```python
from build123d import *

# Parameters (mm, degrees)
SKETCH1_R               = 8
SKETCH1_R_2             = 10
SKETCH1_R_3             = 1.25
SKETCH1_R_4             = 1.5
SKETCH1_R_5             = 1.8
BOSS_EXTRUDE1_DEPTH     = 6
FILLET1_R               = 10
SKETCH2_W               = 15
SKETCH2_H               = 22
BOSS_EXTRUDE2_DEPTH     = 6
SKETCH3_R               = 1
CUT_EXTRUDE1_DEPTH      = 159.031622895
CHAMFER1_SIZE           = 1
MOVE_FACE1_OUTLINE_R    = 8
MOVE_FACE1_OUTLINE_R_2  = 7.92
MOVE_FACE1_OUTLINE_R_3  = 10
MOVE_FACE1_OUTLINE_R_4  = 9.92
MOVE_FACE1_OUTLINE_R_5  = 1.25
MOVE_FACE1_OUTLINE_R_6  = 1.17
MOVE_FACE1_OUTLINE_R_7  = 1.5
MOVE_FACE1_OUTLINE_R_8  = 1.42
MOVE_FACE1_OUTLINE_R_9  = 1.8
MOVE_FACE1_OUTLINE_R_10 = 1.72
MOVE_FACE1_DEPTH        = 6


# Read off the part's stored shape, not the designer's step: Move Face1
with BuildPart() as part:
    # Sketch1 → Boss-Extrude1 (new body)
    with BuildSketch(Plane.XY):
        with BuildLine():
            Line((-40.498784978, 0), (0, 0))
            Line((0, 0), (0, 75))
            ThreePointArc((0, 75), (-37.5, 112.5), (-75, 75))
            Line((-75, 75), (-75, 55))
            Line((-75, 55), (-83.323029145, 55))
            ThreePointArc((-83.323029145, 55), (-110.823029145, 27.5), (-83.323029145, 0))
            Line((-83.323029145, 0), (-40.498784978, 0))
        make_face()
        with Locations((-83.323029145, 27.5)):
            Circle(SKETCH1_R, mode=Mode.SUBTRACT)
        with Locations((-37.5, 75)):
            Circle(SKETCH1_R_2, mode=Mode.SUBTRACT)
        with Locations((-83.323029145, 50.5)):
            Circle(SKETCH1_R_3, mode=Mode.SUBTRACT)
        with Locations((-67.059573177, 43.763455967)):
            Circle(SKETCH1_R_4, mode=Mode.SUBTRACT)
        with Locations((-60.323029145, 27.5)):
            Circle(SKETCH1_R_3, mode=Mode.SUBTRACT)
        with Locations((-67.059573177, 11.236544033)):
            Circle(SKETCH1_R_4, mode=Mode.SUBTRACT)
        with Locations((-83.323029145, 4.5)):
            Circle(SKETCH1_R_3, mode=Mode.SUBTRACT)
        with Locations((-37.5, 102.5)):
            Circle(SKETCH1_R_5, mode=Mode.SUBTRACT)
        with Locations((-65, 75)):
            Circle(SKETCH1_R_5, mode=Mode.SUBTRACT)
        with Locations((-10, 75)):
            Circle(SKETCH1_R_5, mode=Mode.SUBTRACT)
        with Locations((-37.5, 47.5)):
            Circle(SKETCH1_R_5, mode=Mode.SUBTRACT)
        with Locations((-56.945436483, 94.445436483)):
            Circle(SKETCH1_R_4, mode=Mode.SUBTRACT)
        with Locations((-18.054563517, 94.445436483)):
            Circle(SKETCH1_R_4, mode=Mode.SUBTRACT)
        with Locations((-18.054563517, 55.554563517)):
            Circle(SKETCH1_R_4, mode=Mode.SUBTRACT)
        with Locations((-56.945436483, 55.554563517)):
            Circle(SKETCH1_R_4, mode=Mode.SUBTRACT)
        with Locations((-37.5, 88)):
            Circle(SKETCH1_R_5, mode=Mode.SUBTRACT)
        with Locations((-24.5, 75)):
            Circle(SKETCH1_R_5, mode=Mode.SUBTRACT)
        with Locations((-37.5, 62)):
            Circle(SKETCH1_R_5, mode=Mode.SUBTRACT)
        with Locations((-50.5, 75)):
            Circle(SKETCH1_R_5, mode=Mode.SUBTRACT)
    extrude(amount=BOSS_EXTRUDE1_DEPTH)

    # Fillet1
    fillet1_edges = [part.edges().sort_by_distance(p)[0] for p in [
        (-75, 55, 3),
    ]]
    fillet(fillet1_edges, radius=FILLET1_R)

    # Sketch2 → Boss-Extrude2 (add)
    with BuildSketch(Plane(origin=(0, 0, 0), x_dir=(-1, 0, 0), z_dir=(0, 0, -1))):
        with Locations((7.5, -11)):
            Rectangle(SKETCH2_W, SKETCH2_H)
        with Locations((37.5, -11)):
            Rectangle(SKETCH2_W, SKETCH2_H)
        with Locations((67.5, -11)):
            Rectangle(SKETCH2_W, SKETCH2_H)
    extrude(amount=-BOSS_EXTRUDE2_DEPTH)

    # Sketch3 → Cut-Extrude1 (cut, through all)
    with BuildSketch(Plane.XY.offset(6)):
        with Locations((-75, 0)):
            Circle(SKETCH3_R)
        with Locations((-60, 0)):
            Circle(SKETCH3_R)
        with Locations((-45, 0)):
            Circle(SKETCH3_R)
        with Locations((-30, 0)):
            Circle(SKETCH3_R)
        with Locations((-15, 0)):
            Circle(SKETCH3_R)
    extrude(amount=-CUT_EXTRUDE1_DEPTH, mode=Mode.SUBTRACT)

    # Chamfer1
    chamfer1_edges = [part.edges().sort_by_distance(p)[0] for p in [
        (0, -22, 3),
        (-15, -22, 3),
        (-30, -22, 3),
        (-45, -22, 3),
        (-60, -22, 3),
        (-75, -22, 3),
    ]]
    chamfer(chamfer1_edges, length=CHAMFER1_SIZE)

    # Move Face1 outline → Move Face1 (add)
    # profile 1 of 24: a face of its own
    with BuildSketch(Plane.XY):
        with BuildLine():
            Line((-59.003205136, -0.08), (-45.996794864, -0.08))
            ThreePointArc((-45.996794864, -0.08), (-45.999198395, -0.04003209), (-46, 0))
            Line((-46, 0), (-59, 0))
            ThreePointArc((-59, 0), (-59.000801605, -0.04003209), (-59.003205136, -0.08))
        make_face()
    # profile 2 of 24: a face of its own
    with BuildSketch(Plane.XY):
        with BuildLine():
            Line((-45, -21), (-45, -1))
            ThreePointArc((-45, -1), (-45.04003209, -0.999198395), (-45.08, -0.996794864))
            Line((-45.08, -0.996794864), (-45.08, -21.033137085))
            Line((-45.08, -21.033137085), (-44.033137085, -22.08))
            Line((-44.033137085, -22.08), (-30.966862915, -22.08))
            Line((-30.966862915, -22.08), (-29.92, -21.033137085))
            Line((-29.92, -21.033137085), (-29.92, -0.996794864))
            ThreePointArc((-29.92, -0.996794864), (-29.95996791, -0.999198395), (-30, -1))
            Line((-30, -1), (-30, -21))
            Line((-30, -21), (-31, -22))
            Line((-31, -22), (-44, -22))
            Line((-44, -22), (-45, -21))
        make_face()
    # profile 3 of 24: a face of its own
    with BuildSketch(Plane.XY):
        with BuildLine():
            ThreePointArc((-59.92, -0.996794864), (-59.95996791, -0.999198395), (-60, -1))
            Line((-60, -1), (-60, -21))
            Line((-60, -21), (-61, -22))
            Line((-61, -22), (-74, -22))
            Line((-74, -22), (-75, -21))
            Line((-75, -21), (-75, -1))
            ThreePointArc((-75, -1), (-75.04003209, -0.999198395), (-75.08, -0.996794864))
            Line((-75.08, -0.996794864), (-75.08, -21.033137085))
            Line((-75.08, -21.033137085), (-74.033137085, -22.08))
            Line((-74.033137085, -22.08), (-60.966862915, -22.08))
            Line((-60.966862915, -22.08), (-59.92, -21.033137085))
            Line((-59.92, -21.033137085), (-59.92, -0.996794864))
        make_face()
    # profile 4 of 24: a face of its own
    with BuildSketch(Plane.XY):
        with BuildLine():
            Line((-16, 0), (-29, 0))
            ThreePointArc((-29, 0), (-29.000801605, -0.04003209), (-29.003205136, -0.08))
            Line((-29.003205136, -0.08), (-15.996794864, -0.08))
            ThreePointArc((-15.996794864, -0.08), (-15.999198395, -0.04003209), (-16, 0))
        make_face()
    # profile 5 of 24: a face of its own
    with BuildSketch(Plane.XY):
        with BuildLine():
            ThreePointArc((-75.996794864, -0.08), (-75.999198395, -0.04003209), (-76, 0))
            Line((-76, 0), (-83.323029145, 0))
            ThreePointArc((-83.323029145, 0), (-110.816150501, 26.884956844), (-84.552807772, 54.972488867))
            ThreePointArc((-84.552807772, 54.972488867), (-77.772555006, 58.051331596), (-75, 64.962484818))
            Line((-75, 64.962484818), (-75, 75))
            ThreePointArc((-75, 75), (-37.5, 112.5), (0, 75))
            Line((0, 75), (0, -21))
            Line((0, -21), (-1, -22))
            Line((-1, -22), (-14, -22))
            Line((-14, -22), (-15, -21))
            Line((-15, -21), (-15, -1))
            ThreePointArc((-15, -1), (-15.04003209, -0.999198395), (-15.08, -0.996794864))
            Line((-15.08, -0.996794864), (-15.08, -21.033137085))
            Line((-15.08, -21.033137085), (-14.033137085, -22.08))
            Line((-14.033137085, -22.08), (-0.966862915, -22.08))
            Line((-0.966862915, -22.08), (0.08, -21.033137085))
            Line((0.08, -21.033137085), (0.08, 75))
            ThreePointArc((0.08, 75), (-37.5, 112.58), (-75.08, 75))
            Line((-75.08, 75), (-75.08, 64.962484818))
            ThreePointArc((-75.08, 64.962484818), (-77.830374566, 58.106620822), (-84.55638531, 55.052408834))
            ThreePointArc((-84.55638531, 55.052408834), (-110.896130491, 26.883167628), (-83.323029145, -0.08))
            Line((-83.323029145, -0.08), (-75.996794864, -0.08))
        make_face()
    # profile 6 of 24: a face of its own
    with BuildSketch(Plane.XY):
        with Locations((-83.323029145, 27.5)):
            Circle(MOVE_FACE1_OUTLINE_R)
        with Locations((-83.323029145, 27.5)):
            Circle(MOVE_FACE1_OUTLINE_R_2, mode=Mode.SUBTRACT)
    # profile 7 of 24: a face of its own
    with BuildSketch(Plane.XY):
        with Locations((-37.5, 75)):
            Circle(MOVE_FACE1_OUTLINE_R_3)
        with Locations((-37.5, 75)):
            Circle(MOVE_FACE1_OUTLINE_R_4, mode=Mode.SUBTRACT)
    # profile 8 of 24: a face of its own
    with BuildSketch(Plane.XY):
        with Locations((-83.323029145, 50.5)):
            Circle(MOVE_FACE1_OUTLINE_R_5)
        with Locations((-83.323029145, 50.5)):
            Circle(MOVE_FACE1_OUTLINE_R_6, mode=Mode.SUBTRACT)
    # profile 9 of 24: a face of its own
    with BuildSketch(Plane.XY):
        with Locations((-67.059573177, 43.763455967)):
            Circle(MOVE_FACE1_OUTLINE_R_7)
        with Locations((-67.059573177, 43.763455967)):
            Circle(MOVE_FACE1_OUTLINE_R_8, mode=Mode.SUBTRACT)
    # profile 10 of 24: a face of its own
    with BuildSketch(Plane.XY):
        with Locations((-37.5, 102.5)):
            Circle(MOVE_FACE1_OUTLINE_R_9)
        with Locations((-37.5, 102.5)):
            Circle(MOVE_FACE1_OUTLINE_R_10, mode=Mode.SUBTRACT)
    # profile 11 of 24: a face of its own
    with BuildSketch(Plane.XY):
        with Locations((-60.323029145, 27.5)):
            Circle(MOVE_FACE1_OUTLINE_R_5)
        with Locations((-60.323029145, 27.5)):
            Circle(MOVE_FACE1_OUTLINE_R_6, mode=Mode.SUBTRACT)
    # profile 12 of 24: a face of its own
    with BuildSketch(Plane.XY):
        with Locations((-67.059573177, 11.236544033)):
            Circle(MOVE_FACE1_OUTLINE_R_7)
        with Locations((-67.059573177, 11.236544033)):
            Circle(MOVE_FACE1_OUTLINE_R_8, mode=Mode.SUBTRACT)
    # profile 13 of 24: a face of its own
    with BuildSketch(Plane.XY):
        with Locations((-83.323029145, 4.5)):
            Circle(MOVE_FACE1_OUTLINE_R_5)
        with Locations((-83.323029145, 4.5)):
            Circle(MOVE_FACE1_OUTLINE_R_6, mode=Mode.SUBTRACT)
    # profile 14 of 24: a face of its own
    with BuildSketch(Plane.XY):
        with Locations((-65, 75)):
            Circle(MOVE_FACE1_OUTLINE_R_9)
        with Locations((-65, 75)):
            Circle(MOVE_FACE1_OUTLINE_R_10, mode=Mode.SUBTRACT)
    # profile 15 of 24: a face of its own
    with BuildSketch(Plane.XY):
        with Locations((-10, 75)):
            Circle(MOVE_FACE1_OUTLINE_R_9)
        with Locations((-10, 75)):
            Circle(MOVE_FACE1_OUTLINE_R_10, mode=Mode.SUBTRACT)
    # profile 16 of 24: a face of its own
    with BuildSketch(Plane.XY):
        with Locations((-37.5, 47.5)):
            Circle(MOVE_FACE1_OUTLINE_R_9)
        with Locations((-37.5, 47.5)):
            Circle(MOVE_FACE1_OUTLINE_R_10, mode=Mode.SUBTRACT)
    # profile 17 of 24: a face of its own
    with BuildSketch(Plane.XY):
        with Locations((-56.945436483, 94.445436483)):
            Circle(MOVE_FACE1_OUTLINE_R_7)
        with Locations((-56.945436483, 94.445436483)):
            Circle(MOVE_FACE1_OUTLINE_R_8, mode=Mode.SUBTRACT)
    # profile 18 of 24: a face of its own
    with BuildSketch(Plane.XY):
        with Locations((-37.5, 88)):
            Circle(MOVE_FACE1_OUTLINE_R_9)
        with Locations((-37.5, 88)):
            Circle(MOVE_FACE1_OUTLINE_R_10, mode=Mode.SUBTRACT)
    # profile 19 of 24: a face of its own
    with BuildSketch(Plane.XY):
        with Locations((-18.054563517, 94.445436483)):
            Circle(MOVE_FACE1_OUTLINE_R_7)
        with Locations((-18.054563517, 94.445436483)):
            Circle(MOVE_FACE1_OUTLINE_R_8, mode=Mode.SUBTRACT)
    # profile 20 of 24: a face of its own
    with BuildSketch(Plane.XY):
        with Locations((-18.054563517, 55.554563517)):
            Circle(MOVE_FACE1_OUTLINE_R_7)
        with Locations((-18.054563517, 55.554563517)):
            Circle(MOVE_FACE1_OUTLINE_R_8, mode=Mode.SUBTRACT)
    # profile 21 of 24: a face of its own
    with BuildSketch(Plane.XY):
        with Locations((-56.945436483, 55.554563517)):
            Circle(MOVE_FACE1_OUTLINE_R_7)
        with Locations((-56.945436483, 55.554563517)):
            Circle(MOVE_FACE1_OUTLINE_R_8, mode=Mode.SUBTRACT)
    # profile 22 of 24: a face of its own
    with BuildSketch(Plane.XY):
        with Locations((-24.5, 75)):
            Circle(MOVE_FACE1_OUTLINE_R_9)
        with Locations((-24.5, 75)):
            Circle(MOVE_FACE1_OUTLINE_R_10, mode=Mode.SUBTRACT)
    # profile 23 of 24: a face of its own
    with BuildSketch(Plane.XY):
        with Locations((-37.5, 62)):
            Circle(MOVE_FACE1_OUTLINE_R_9)
        with Locations((-37.5, 62)):
            Circle(MOVE_FACE1_OUTLINE_R_10, mode=Mode.SUBTRACT)
    # profile 24 of 24: a face of its own
    with BuildSketch(Plane.XY):
        with Locations((-50.5, 75)):
            Circle(MOVE_FACE1_OUTLINE_R_9)
        with Locations((-50.5, 75)):
            Circle(MOVE_FACE1_OUTLINE_R_10, mode=Mode.SUBTRACT)
    extrude(amount=MOVE_FACE1_DEPTH)


solid = part.part
```
Can you work these out from the model? Positions are in its coordinate system, mm. A direction names the side the tool comes from. Round coordinates to 2 decimals unless told otherwise and drop trailing zeros. Loops run counter-clockwise (first coordinate to the right, second up) from the corner with the lowest first, then second, coordinate; pieces in that order, holes last. Notation, with made-up numbers: (75.5, -29.75) -> (116.5, -29.75) arc R20 ccw to (116.5, -21.75) -> close; hole circle Ø5 at (-22.75, 33). An arc over 180 degrees is marked (long way). One line per item, written item: value. Start each with the question number.
1. If we section it at B-B, the plane y = 102.5: Write out the boundary of the cut face in (x, z), then the cut area to 3 significant figures.
2. If we section it at D-D, the plane z = 4.8: Give the number of separate pieces and of enclosed holes in the cut face, then the cut area to 3 significant figures.
3. If I drill on probe 1 along Y at (x, z) = (-37.5, 1.2); probe 2 along X at (y, z) = (-4.5, 0.5); probe 3 along X at (y, z) = (27, 2), over which ranges is the centre line in solid material (lowest first)?
4. For pin 1 (2.5 mm diameter, centred on x = -67.06, y = 43.76, fed in from -Z); pin 2 (1.5 mm diameter, centred on y = 39.5, z = 1, fed in from -X); pin 3 (1 mm diameter, centred on x = -90.5, z = 2.5, fed in from +Y); pin 4 (1.5 mm diameter, centred on y = 76.5, z = 0.5, fed in from -X), each with a flat end and sliding along its axis, tell me the tip position at first contact or that it passes through.
5. For faces 1 (the cylindrical face through (-49.71, 73.47, 2.96)), 2 (the flat face through (-75.08, -11, 3)), 3 (the flat face through (-53, -0.08, 3)), which set-ups out of +Z, -Z, +X, -X, +Y, -Y let a thin tool reach every point of the face, with its end or its side?
6. If we section it at C-C, the plane x = -89.5: Write out the boundary of the cut face in (y, z), then the cut area to 3 significant figures.
7. If we section it at A-A, the plane x = -37.5: Write out the boundary of the cut face in (y, z).
8. If we mould it in two halves opening along Y, with no side actions, what happens to faces 4 (the flat face through (-80, -0.08, 3)), 5 (the cylindrical face through (-89.608, 22.681, 2.958)), 6 (the flat face through (-44, 46, 6))? For each: pulls with the +Y half, pulls with the -Y half, needs draft (parallel to the pull), parting line crosses it, or undercut.
Calculated:
1. outline: (-63.11, 0) -> (-39.22, 0) -> (-39.22, 6) -> (-63.11, 6) -> close; (-35.78, 0) -> (-11.89, 0) -> (-11.89, 6) -> (-35.78, 6) -> close
1. area: 287 mm²
2. separate pieces: 1
2. enclosed holes: 19
2. area: 9,880 mm²
3. probe 1: y = -22.08 to 45.78, 49.22 to 60.28, 63.72 to 65.08, 84.92 to 86.28, 89.72 to 100.78, 104.22 to 112.58
3. probe 2: x = -75.08 to -59.92, -45.08 to -29.92, -15.08 to 0.08
3. probe 3: x = -110.9 to -91.23, -75.42 to -61.38, -59.27 to 0.08
4. pin 1: passes through
4. pin 2: stops at x = -108.5
4. pin 3: stops at y = 54.26
4. pin 4: stops at x = -75.07
5. face 1: +Z, -Z
5. face 2: +Z, -Z, -X, -Y
5. face 3: +Z, -Z, -Y
6. outline: (0.62, 0) -> (22.54, 0) -> (22.54, 6) -> (0.62, 6) -> close; (32.46, 0) -> (54.38, 0) -> (54.38, 6) -> (32.46, 6) -> close
6. area: 263 mm²
7. outline: (-22.08, 0) -> (45.78, 0) -> (45.78, 6) -> (-22.08, 6) -> close; (49.22, 0) -> (60.28, 0) -> (60.28, 6) -> (49.22, 6) -> close; (63.72, 0) -> (65.08, 0) -> (65.08, 6) -> (63.72, 6) -> close; (84.92, 0) -> (86.28, 0) -> (86.28, 6) -> (84.92, 6) -> close; (89.72, 0) -> (100.78, 0) -> (100.78, 6) -> (89.72, 6) -> close; (104.22, 0) -> (112.58, 0) -> (112.58, 6) -> (104.22, 6) -> close
8. face 4: pulls with the -Y half
8. face 5: undercut
8. face 6: needs draft
